Geometry: see drawing. Coordinates: mm, zero at the bounding-box minimum. Coordinates: 2 decimals unless noted, no trailing zeros. Order: outer loops, then holes, each group sorted by start corner. A loop starts at its lowest first (then second) coordinate and runs counter-clockwise, first axis right, second up.
Item 1: Section C-C on x = 189. Return the cut outline in (y, z), then the cut area to 3 significant figures.
Item 2: Mould query, pull axis X, two halves, no side actions, for the marked faces 1 and 2. Classes: released by +X, released by -X, zero draft, split by the parting line, or undercut.
Item 3: Section A-A on y = 19.75. Return the cut outline in (x, z).
Item 4: Ray query, line 1 (X direction, y = 20, z = 287); line 2 (Z direction, x = 226, y = 13.25); line 3 (Y direction, x = 176, z = 214.5). Return the intervals inside material, ascending.
Item 5: Section B-B on z = 195. Return the cut outline in (x, y).
Item 6: Contact query for a flat-ended pin moving along its axis: P1, Ø12, axis at x = 158.5, z = 391, coming from the +Y side. Output: stop coordinate, or through.
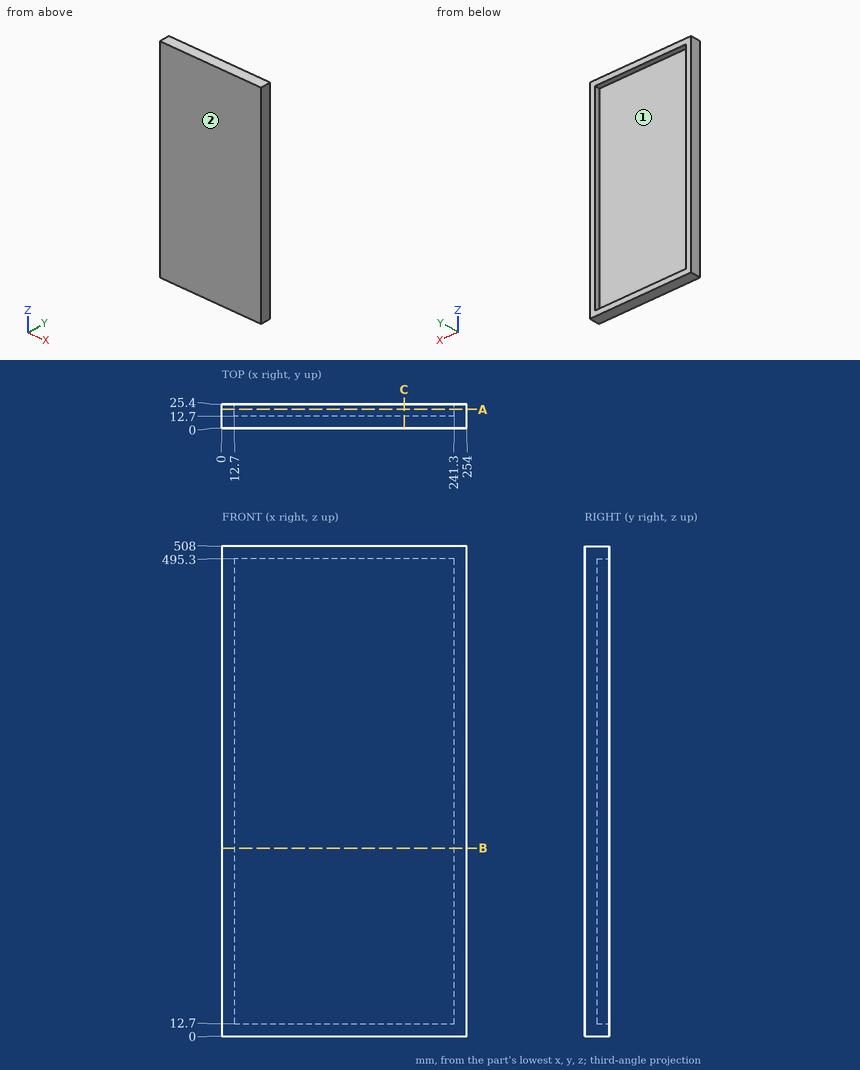
Answer list:
1. outline: (0, 0) - (25.4, 0) - (25.4, 12.7) - (12.7, 12.7) - (12.7, 495.3) - (25.4, 495.3) - (25.4, 508) - (0, 508) - close
1. area: 6,770 mm2
2. face 1: undercut
2. face 2: zero draft
3. outline: (0, 0) - (254, 0) - (254, 508) - (0, 508) - close; hole (12.7, 12.7) - (241.3, 12.7) - (241.3, 495.3) - (12.7, 495.3) - close
4. line 1: x = 0 to 12.7, 241.3 to 254
4. line 2: z = 0 to 12.7, 495.3 to 508
4. line 3: y = 0 to 12.7
5. outline: (0, 0) - (254, 0) - (254, 25.4) - (241.3, 25.4) - (241.3, 12.7) - (12.7, 12.7) - (12.7, 25.4) - (0, 25.4) - close
6. P1: stops at y = 12.7
